Design review of the part shown in the three views and the two pictorial views. Dimensions are in mm from the part's minimum x, y and z. A direction names the side the tool comes from. Give positions to 0.01 mm unless a question says otherwise; leave off trailing zeros. Order: outer loops, then holes, each group sorted by start corner. A loop starts at its lowest first (then second) coordinate and runs counter-clockwise, first axis right, second up. Notation, with made-up numbers: (4, 43.5) - (45, 43.5) arc R15 cw to (45, 55.5) - close; hole circle Ø1 at (30.5, 63.5). An arc over 180 degrees is marked (long way). Put each result on its own line as item: value. Start each with the question number.
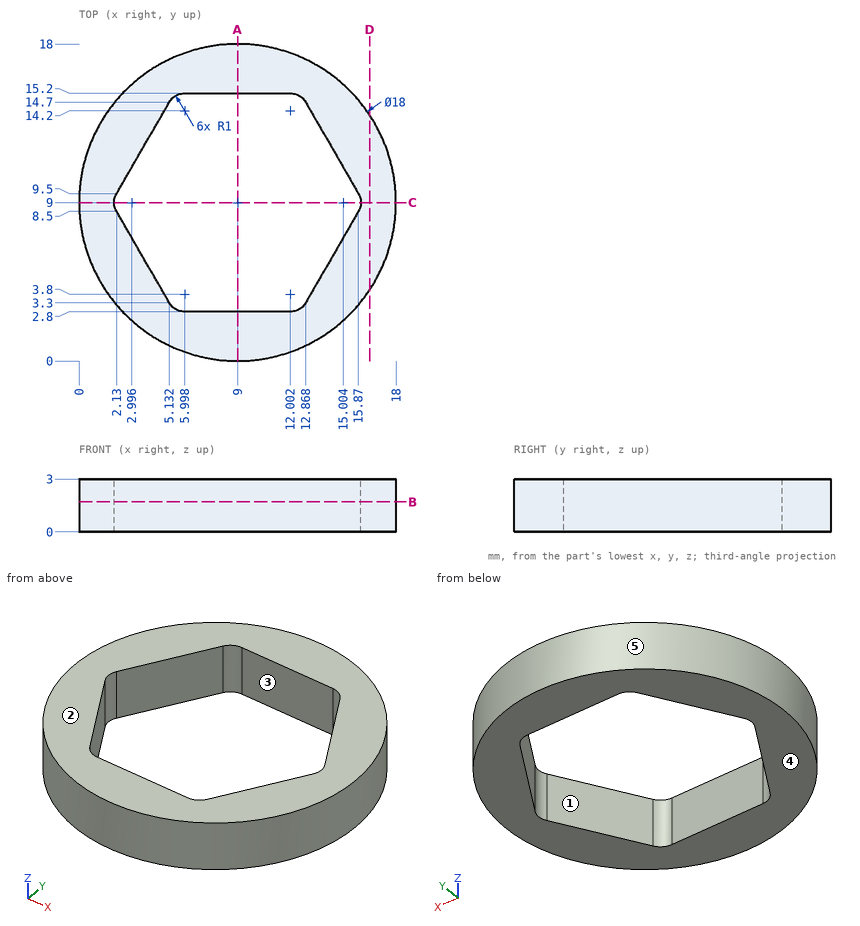
1. Wall thickness on line 1 (Y direction, x = 9.25, z = 2.15); line 2 (X direction, y = 6.5, z = 0.8) (1 decimal); line 3 (Y direction, x = 10.5, z = 1.7) (1 decimal): over which ranges is each line inside the solid? List them lowest first. Write a range as from..to.
2. The part is to be moulded in two halves that separate along X. For the marked faces 3, 4 and 5, say which applies: released by +X, released by -X, zero draft, split by the parting line, or undercut.
3. Add section C-C, the plane y = 9. Give the boundary of the cut face in (x, z) (1 decimal), then the cut area to 3 significant figures.
4. Tool access review of the marked faces 1 and 2: name each direction out of +Z, -Z, +X, -X, +Y, -Y from which nothing blocks a thin tool from reaching the whole face with its end or side.
5. Add section A-A, the plane x = 9. Give the boundary of the cut face in (y, z), then the cut area to 3 significant figures.
6. Clearance check with flat-ended pins moving along their axes: pin 1 (1.5 mm diameter, centred on y = 4.5, z = 1, fed in from +X); pin 2 (1 mm diameter, centred on y = 6.5, z = 1.5, fed in from +X) (1 decimal); pin 3 (1 mm diameter, centred on y = 3, z = 0.5, fed in from -X) (1 decimal). State where each tip first meets the part, or that it passes through.
7. Add section D-D, the plane x = 16.5. Give the boundary of the cut face in (y, z) (1 decimal).
8. Add section B-B, the plane z = 1.7. Give the boundary of the cut face in (x, y) (1 decimal).
Found:
1. line 1: y = 0..2.8, 15.2..18
1. line 2: x = 0.4..3.3, 14.7..17.6
1. line 3: y = 0.1..2.8, 15.2..17.9
2. face 3: undercut
2. face 4: zero draft
2. face 5: split by the parting line
3. outline: (0, 0) - (2, 0) - (2, 3) - (0, 3) - close; (16, 0) - (18, 0) - (18, 3) - (16, 3) - close
3. area: 12.0 mm^2
4. face 1: +Z, -Z
4. face 2: +Z, +X, -X, +Y, -Y
5. outline: (0, 0) - (2.8, 0) - (2.8, 3) - (0, 3) - close; (15.2, 0) - (18, 0) - (18, 3) - (15.2, 3) - close
5. area: 16.8 mm^2
6. pin 1: stops at x = 17.18
6. pin 2: stops at x = 17.8
6. pin 3: stops at x = 1.9
7. outline: (4, 0) - (14, 0) - (14, 3) - (4, 3) - close
8. outline: circle Ø18 at (9, 9); hole (2.1, 8.5) - (5.1, 3.3) arc R1 ccw to (6, 2.8) - (12, 2.8) arc R1 ccw to (12.9, 3.3) - (15.9, 8.5) arc R1 ccw to (15.9, 9.5) - (12.9, 14.7) arc R1 ccw to (12, 15.2) - (6, 15.2) arc R1 ccw to (5.1, 14.7) - (2.1, 9.5) arc R1 ccw to start
